Work out the finished part from the listing and answer in its coordinate system (mm). Face numbers are marked on the shaded views. A direction names the side the tool comes from. Coordinates: 2 decimals unless noted, no trailing zeros. Loops run counter-clockwise (first coordinate to the right, second up) from the corner with the lowest first, then second, coordinate; pieces in that order, holes last. Notation, with made-up numbers: (77.5, 77.25) -> (123.5, 77.25) arc R20 ccw to (123.5, 108.25) -> close; hole circle Ø4 at (2, -15). An arc over 180 degrees is marked (long way). One line per question, with ' | ' between items.
```python
from build123d import *

# Parameters (mm, degrees)
F1_DEPTH  = 16
F2_W      = 70
F2_H      = 3
F3_DEPTH  = 2
F4_W      = 50
F4_H      = 12
F5_DEPTH  = 2
F6_R      = 1
F9_DEPTH  = 2
F11_DEPTH = 38.001
F13_D     = 4
F14_R     = 3
F14_R_2   = 2
F15_DEPTH = 5


# Not quite as in the source:
# - a pattern or mirror of a feature is missing from the dataset's text; its kind, count and spacing are read off the source's solid


with BuildPart() as f1:
    # F0 (on Front) → F1 (new body)
    with BuildSketch(Plane.XZ):
        with BuildLine():
            Line((46.2855722755, 5.7414249778), (-47.7144277245, 5.7414249778))
            ThreePointArc((-47.7144277245, 5.7414249778), (-58.7144277245, -5.2585750222), (-47.7144277245, -16.2585750222))
            Line((-47.7144277245, -16.2585750222), (-28.7144277245, -16.2585750222))
            ThreePointArc((-28.7144277245, -16.2585750222), (-25.7968307423, -17.5210599177), (-24.7197856057, -20.5120821569))
            ThreePointArc((-24.7197856057, -20.5120821569), (-0.5386319719, -49.8206199667), (35.0020481502, -63.2585750222))
            ThreePointArc((35.0020481502, -63.2585750222), (39.8678360266, -64.6074545818), (44.1721712505, -67.2471640366))
            Line((44.1721712505, -67.2471640366), (45.9107602648, -66.2585750222))
            ThreePointArc((45.9107602648, -66.2585750222), (40.9429054682, -62.6971545828), (35.0020481502, -61.2585750222))
            ThreePointArc((35.0020481502, -61.2585750222), (0.6230450398, -48.7022972109), (-22.7197856057, -20.5120821569))
            ThreePointArc((-22.7197856057, -20.5120821569), (-24.3830859689, -16.1065299122), (-28.7144277245, -14.2585750222))
            Line((-28.7144277245, -14.2585750222), (-47.7144277245, -14.2585750222))
            ThreePointArc((-47.7144277245, -14.2585750222), (-56.7144277245, -5.2585750222), (-47.7144277245, 3.7414249778))
            Line((-47.7144277245, 3.7414249778), (46.2855722755, 3.7414249778))
            Line((46.2855722755, 3.7414249778), (46.2855722755, 5.7414249778))
        make_face()
    extrude(amount=F1_DEPTH)

    # F2 (on face) → F3 (join)
    with BuildSketch(Plane.XY.offset(5.7414249778)):
        with Locations((11.2855722755, -17.5)):
            Rectangle(F2_W, F2_H)
    extrude(amount=-F3_DEPTH)

    # F4 (on face) → F5 (join)
    with BuildSketch(Plane.XZ.offset(19)):
        with Locations((21.2855722755, -2.2585750222)):
            Rectangle(F4_W, F4_H)
    extrude(amount=-F5_DEPTH)

    # F6
    f6_edges = [f1.edges().sort_by_distance(p)[0] for p in [
        (11.285572, -19, 5.741425),
        (21.285572, -17, 3.741425),
    ]]
    fillet(f6_edges, radius=F6_R)

    # F7: F1 across plane


with BuildPart() as f1_1:
    add(f1.part)
    add(f1.part.mirror(Plane.XZ))

    # F8 (on face) → F9 (cut)
    with BuildSketch(Plane.XY.offset(5.7414249778)):
        with BuildLine():
            Line((46.2855722755, 12), (-13.7144277245, 12))
            ThreePointArc((-13.7144277245, 12), (-25.7144277245, 0), (-13.7144277245, -12))
            Line((-13.7144277245, -12), (46.2855722755, -12))
            Line((46.2855722755, -12), (46.2855722755, 12))
        make_face()
    extrude(amount=-F9_DEPTH, mode=Mode.SUBTRACT)

    # F10 (on face) → F11 (cut, through all)
    with BuildSketch(Plane.XZ.offset(19)):
        with BuildLine():
            ThreePointArc((2.2855722755, -0.2585750222), (-0.7144277245, -3.2585750222), (2.2855722755, -6.2585750222))
            Line((2.2855722755, -6.2585750222), (22.2855722755, -6.2585750222))
            ThreePointArc((22.2855722755, -6.2585750222), (25.2855722755, -3.2585750222), (22.2855722755, -0.2585750222))
            Line((22.2855722755, -0.2585750222), (2.2855722755, -0.2585750222))
        make_face()
    extrude(amount=-F11_DEPTH, mode=Mode.SUBTRACT)

    # F13 (through all)
    with Locations(Plane.XZ.offset(19)):
        with Locations((32.2855722755, -2.2585750222)):
            Hole(F13_D / 2)

    # F14 (on face) → F15 (join)
    with BuildSketch(Plane(origin=(0, -17, 0), x_dir=(-1, 0, 0), z_dir=(0, 1, 0))):
        with Locations((-32.2855722755, -2.2585750222)):
            Circle(F14_R)
        with Locations((-32.2855722755, -2.2585750222)):
            Circle(F14_R_2, mode=Mode.SUBTRACT)
    f15 = extrude(amount=F15_DEPTH)

    # F15_copies: F15 across plane
    add(f15.mirror(Plane.ZX))


solid = f1_1.part
```
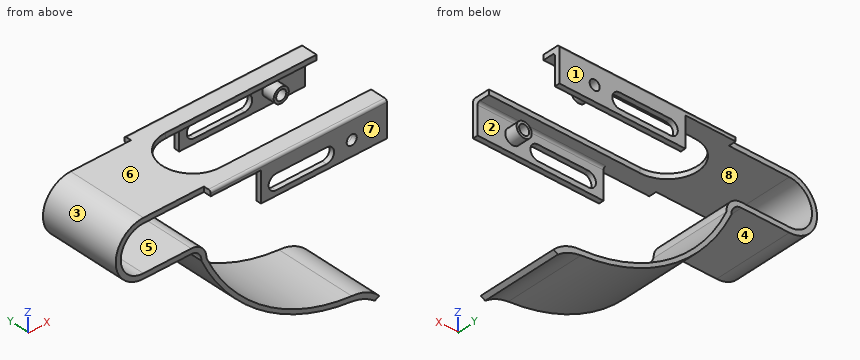
1) The mould has two halves that part along Y. Classify the marked faces 1, 2 and 3: released by +Y, released by -Y, zero draft, split by the parting line, or undercut.
Check values:
face 1: released by +Y | face 2: undercut | face 3: zero draft
2) For the marked faces 4, 5, 6, 7 and 8, determine the directions among +Z, -Z, +X, -X, +Y, -Y from which every point of the face is accessible in a straight line to the end or side of a thin tool.
Check values:
face 4: -Z, -X, +Y, -Y | face 5: +X, +Y, -Y | face 6: +Z, +X, -X, +Y, -Y | face 7: +Z, -Z, +X, -X, -Y | face 8: none
3) Find the intervals of material crossed by line 1 along Z through (x, y) = (-42.5, -6); line 2 along Z through (x, y) = (21, 17.5); line 3 along Y through (x, z) = (12.5, -6.5), in increasing order.
Check values:
line 1: z = -16.26 to -14.26, 3.74 to 5.74 | line 2: z = -8.26 to -6.26, -0.26 to 5.74 | line 3: y = -19 to -17, 17 to 19
4) Find section B-B (y = 0). Write down the section's boundary in (x, z).
Check values:
outline: (-47.71, -16.26) -> (-28.71, -16.26) arc R4 cw to (-24.72, -20.51) arc R73.97 ccw to (35, -63.26) arc R18.11 cw to (44.17, -67.25) -> (45.91, -66.26) arc R16 ccw to (35, -61.26) arc R70 cw to (-22.72, -20.51) arc R6 ccw to (-28.71, -14.26) -> (-47.71, -14.26) arc R9 cw to (-47.71, 3.74) -> (-25.71, 3.74) -> (-25.71, 5.74) -> (-47.71, 5.74) arc R11 ccw to start
5) Find section D-D (x = 21). Write down the section's boundary in (y, z).
Check values:
outline: (-19, -8.26) -> (-17, -8.26) -> (-17, -6.26) -> (-19, -6.26) -> close; (-19, -0.26) -> (-17, -0.26) -> (-17, 2.74) arc R1 cw to (-16, 3.74) -> (-12, 3.74) -> (-12, 5.74) -> (-18, 5.74) arc R1 ccw to (-19, 4.74) -> close; (-16, -60.44) -> (16, -60.44) -> (16, -58.6) -> (-16, -58.6) -> close; (12, 3.74) -> (16, 3.74) arc R1 cw to (17, 2.74) -> (17, -0.26) -> (19, -0.26) -> (19, 4.74) arc R1 ccw to (18, 5.74) -> (12, 5.74) -> close; (17, -8.26) -> (19, -8.26) -> (19, -6.26) -> (17, -6.26) -> close
6) Flat-ended cylindrical pins translate along their axes: pin 1 (0.9 mm diameter, centred on y = 17, z = -1.5, fed in from -X); pin 2 (6 mm diameter, centred on y = 1, z = -2, fed in from -X); pin 3 (2 mm diameter, centred on y = -5, z = -14, fed in from +X); pin 4 (12 mm diameter, centred on x = -13, z = -6.5, fed in from -Y). Find the tip coordinate at first contact, or state that the pin passes through.
Check values:
pin 1: stops at x = -3.71 | pin 2: stops at x = -58.71 | pin 3: stops at x = -25.83 | pin 4: passes through
7) Find section C-C (x = -15). Write down the section's boundary in (y, z).
Check values:
outline: (-19, 3.74) -> (-11.93, 3.74) -> (-11.93, 5.74) -> (-18, 5.74) arc R1 ccw to (-19, 4.74) -> close; (-16, -36.19) -> (16, -36.19) -> (16, -33.53) -> (-16, -33.53) -> close; (11.93, 3.74) -> (19, 3.74) -> (19, 4.74) arc R1 ccw to (18, 5.74) -> (11.93, 5.74) -> close
8) Find section A-A (x = -44). Write down the section's boundary in (y, z).
Check values:
outline: (-16, -16.26) -> (16, -16.26) -> (16, -14.26) -> (-16, -14.26) -> close; (-16, 3.74) -> (16, 3.74) -> (16, 5.74) -> (-16, 5.74) -> close
